Build history of the part. All positions in model axes, mm. Face numbers are marked on the shaded views. A direction names the side the tool comes from. Round coordinates to 2 decimals unless told otherwise and drop trailing zeros. Order: outer loops, then holes, each group sorted by start corner. A loop starts at its lowest first (then second) coordinate and runs counter-clockwise, first axis right, second up. Notation, with made-up numbers: M -38.5,-20.75 L -27.5,-20.75 A31 ccw -27.5,14.25 Z; hole C -35.5,-38.75 d11. An arc over 180 degrees is marked long. Use CSV: the item, a comma, the result in double quotes.
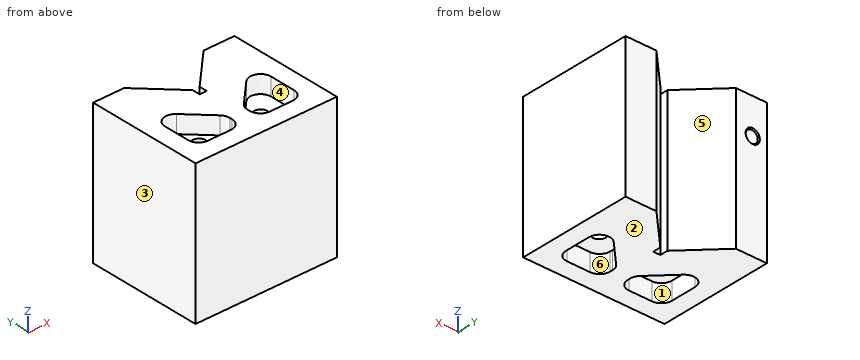
from build123d import *

# Parameters (mm, degrees)
Y_KSEKLIK_EKSTR_ZYON1_DEPTH = 40
IZIM2_R                     = 3.75
KES_EKSTR_ZYON1_DEPTH       = 10
IZIM3_R                     = 3.75
KES_EKSTR_ZYON2_DEPTH       = 81
M8_DI_LI_DELIK1_D           = 6.8
M8_DI_LI_DELIK1_DEPTH       = 18
M8_DI_LI_DELIK1_CSINK_D     = 8.05
M8_DI_LI_DELIK1_CSINK_ANGLE = 90
M8_DI_LI_DELIK1_TIP         = 2.042926105


with BuildPart() as part:
    # Çizim1 → Yükseklik-Ekstrüzyon1 (new body, symmetric)
    with BuildSketch(Plane.XY):
        Polygon((2, 0), (-2, 0), (-2, 4.5), (-22.5, 25), (-40, 25), (-40, -40), (40, -40), (40, 25), (22.5, 25), (2, 4.5), align=None)
    extrude(amount=Y_KSEKLIK_EKSTR_ZYON1_DEPTH, both=True)

    # Çizim2 → Kes-Ekstrüzyon1 (cut)
    with BuildSketch(Plane.XY.offset(40)):
        with BuildLine():
            Line((30, -9.485281374), (30, -24))
            ThreePointArc((30, -24), (28.242640687, -28.242640687), (24, -30))
            Line((24, -30), (11, -30))
            ThreePointArc((11, -30), (6.757359313, -28.242640687), (5, -24))
            Line((5, -24), (5, -22.485281374))
            ThreePointArc((5, -22.485281374), (5.456722805, -20.18918078), (6.757359313, -18.242640687))
            Line((6.757359313, -18.242640687), (19.757359313, -5.242640687))
            ThreePointArc((19.757359313, -5.242640687), (26.296100594, -3.942004179), (30, -9.485281374))
        make_face()
        with Locations((17.5, -17)):
            Circle(IZIM2_R, mode=Mode.SUBTRACT)
        with BuildLine():
            Line((-24, -30), (-11, -30))
            ThreePointArc((-11, -30), (-6.757359313, -28.242640687), (-5, -24))
            Line((-5, -24), (-5, -22.485281374))
            ThreePointArc((-5, -22.485281374), (-5.456722805, -20.18918078), (-6.757359313, -18.242640687))
            Line((-6.757359313, -18.242640687), (-19.757359313, -5.242640687))
            ThreePointArc((-19.757359313, -5.242640687), (-26.296100594, -3.942004179), (-30, -9.485281374))
            Line((-30, -9.485281374), (-30, -24))
            ThreePointArc((-30, -24), (-28.242640687, -28.242640687), (-24, -30))
        make_face()
        with Locations((-17.5, -17)):
            Circle(IZIM2_R, mode=Mode.SUBTRACT)
    kes_ekstr_zyon1 = extrude(amount=-KES_EKSTR_ZYON1_DEPTH, mode=Mode.SUBTRACT)

    # Aynalama1: Kes-Ekstrüzyon1 across plane
    add(kes_ekstr_zyon1.mirror(Plane.XY), mode=Mode.SUBTRACT)

    # Çizim3 → Kes-Ekstrüzyon2 (cut, through all)
    with BuildSketch(Plane.XY.offset(40)):
        with Locations((-17.5, -17)):
            Circle(IZIM3_R)
        with Locations((17.5, -17)):
            Circle(IZIM3_R)
    extrude(amount=-KES_EKSTR_ZYON2_DEPTH, mode=Mode.SUBTRACT)

    # M8 Dişli Delik1
    with Locations(Plane(origin=(0, 25, 0), x_dir=(1, 0, 0), z_dir=(0, 1, 0))):
        with Locations((-32, -20)):
            CounterSinkHole(M8_DI_LI_DELIK1_D / 2, M8_DI_LI_DELIK1_CSINK_D / 2, depth=M8_DI_LI_DELIK1_DEPTH, counter_sink_angle=M8_DI_LI_DELIK1_CSINK_ANGLE)
            with Locations((0, 0, -(M8_DI_LI_DELIK1_DEPTH + M8_DI_LI_DELIK1_TIP / 2))):  # 118° drill point
                Cone(0, M8_DI_LI_DELIK1_D / 2, M8_DI_LI_DELIK1_TIP, mode=Mode.SUBTRACT)


solid = part.part
(1) Cut at A-A, the plane y = 13. Give the cut face in (x, z).
Answer block:
outline,"M -40,-40 L -10.5,-40 L -10.5,40 L -40,40 Z; M 10.5,-40 L 40,-40 L 40,40 L 10.5,40 Z; hole C -32,20 d6.8"
(2) Drop flat-ended pins along their axis: pin 1 (3 mm diameter, centred on x = -16, z = -35.5, fed in from +Y); pin 2 (3 mm diameter, centred on x = -14.5, z = 37.5, fed in from +Y); pin 3 (6 mm diameter, centred on x = 17.5, y = -17, fed in from +Z); pin 4 (5 mm diameter, centred on x = 18, z = -33.5, fed in from +Y). Give the stop position or say it passes through.
Answer block:
pin 1,"stops at y = 20"
pin 2,"stops at y = 18.5"
pin 3,"passes through"
pin 4,"stops at y = 23"
(3) Wall check: line 1 (X direction, y = 3, z = 25); line 2 (Z direction, x = -32, y = 19.25); line 3 (X direction, y = 18.5, z = 20). Give the ranges that are in metal, low to high. Write a range as from..to.
Answer block:
line 1,"x = -40..-2, 2..40"
line 2,"z = -40..16.6, 23.4..40"
line 3,"x = -40..-35.4, -28.6..-16, 16..40"
(4) Cut at D-D, the plane z = -14. Give the cut face in (x, y).
Answer block:
outline,"M -40,-40 L 40,-40 L 40,25 L 22.5,25 L 2,4.5 L 2,0 L -2,0 L -2,4.5 L -22.5,25 L -40,25 Z; hole C -17.5,-17 d7.5; hole C 17.5,-17 d7.5"
(5) Tool access for the marked faces 4, 5 and 6: list every direction of +Z, -Z, +X, -X, +Y, -Y with a clear straight run to the whole face (end or side of a thin tool).
Answer block:
face 4,"+Z"
face 5,"+Z, -Z, +Y"
face 6,"-Z"
(6) Two-plate mould, pull along X, no slides. Class the marked faces 1, 2 and 3: released by +X, released by -X, zero draft, split by the parting line, or undercut.
Answer block:
face 1,"undercut"
face 2,"zero draft"
face 3,"released by -X"
(7) Cut at C-C, the plane y = -17. Give the cut face in (x, z), and give its area (3 significant figures).
Answer block:
outline,"M -40,-40 L -30,-40 L -30,-30 L -21.25,-30 L -21.25,30 L -30,30 L -30,40 L -40,40 Z; M -13.75,-30 L -8,-30 L -8,-40 L 8,-40 L 8,-30 L 13.75,-30 L 13.75,30 L 8,30 L 8,40 L -8,40 L -8,30 L -13.75,30 Z; M 21.25,-30 L 30,-30 L 30,-40 L 40,-40 L 40,40 L 30,40 L 30,30 L 21.25,30 Z"
area,"4,620 mm²"
(8) Cut at B-B, the plane x = 17.5. Give the cut face in (y, z), and give its area (3 significant figures).
Answer block:
outline,"M -40,-40 L -30,-40 L -30,-30 L -20.75,-30 L -20.75,30 L -30,30 L -30,40 L -40,40 Z; M -13.25,-30 L -7.5,-30 L -7.5,-40 L 20,-40 L 20,40 L -7.5,40 L -7.5,30 L -13.25,30 Z"
area,"3,900 mm²"
